Geometry check sheet. Reference: the model listing, model coordinates, mm. Face numbers are marked on the shaded views. Coordinates: 2 decimals unless noted, no trailing zeros. Write each loop counter-clockwise with the first axis right and the second up, starting at its lowest first coordinate (ties: lowest second). Pieces come first, ordered by that corner, then holes. Notation, with made-up numbers: (-18, 55) -> (3, 55) arc R23 cw to (3, 79) -> close; hole circle Ø8 at (21, 69.5). An arc over 180 degrees is marked (long way). Answer in a Markdown table with one row per item. Add a question column.
Q1. Section check A-A, the plane z = 5.25. Record the boundary of the cut face in (x, y), and give its area (3 significant figures).
Q2. Section check C-C, the plane x = 0.25. Record the boundary of the cut face in (y, z), and give its area (3 significant figures).
Q3. Gauge pin test, flat ends, axial feed: P1, Ø5, axis at x = 0, y = 0, coming from the -Z side; P2, Ø5, axis at x = 3, z = 6, coming from the -Y side; P3, Ø1.5, axis at x = 3, z = 3.5, coming from the -Y side. Record the tip position at first contact, or that the pin passes through.
Q4. Release check for a two-part mould opening along Y. For the marked faces 1, 2, 3 and 4 record: pulls with the +Y half, pulls with the -Y half, needs draft (parallel to the pull), parting line crosses it, or undercut.
Q5. Section check D-D, the plane x = -2.25. Record the boundary of the cut face in (y, z), and give its area (3 significant figures).
Q6. Thickness scan on line 1 (X direction, y = 0, z = 7.5); line 2 (X direction, y = 0, z = 3); line 3 (Z direction, x = 2.75, y = 2.25). Record the ranges inside material, lowest first.
Q7. Section check B-B, the plane y = 0. Record the boundary of the cut face in (x, z), and give its area (3 significant figures).
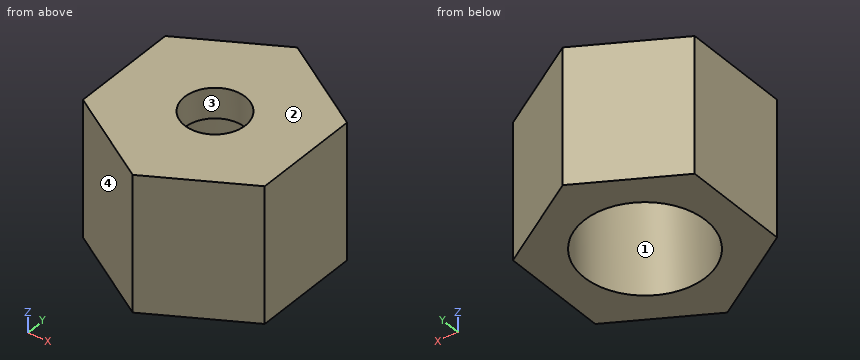
Autodesk Inventor part; units mm, degrees
ref_plane "YZ Plane" through (0, 0, 0) normal (1, 0, 0) x (0, 1, 0)
ref_plane "XZ Plane" through (0, 0, 0) normal (0, 1, 0) x (-1, 0, 0)
ref_plane "XY Plane" through (0, 0, 0) normal (0, 0, 1) x (1, 0, 0)
sketch "Sketch1" plane through (0, 0, 0) normal (0, 0, 1) x (1, 0, 0)
  line L0 (0, -6.9282) -> (-6, -3.4641)
  line L1 (-6, -3.4641) -> (-6, 3.4641)
  line L2 (-6, 3.4641) -> (0, 6.9282)
  line L3 (0, 6.9282) -> (6, 3.4641)
  line L4 (6, 3.4641) -> (6, -3.4641)
  line L5 (6, -3.4641) -> (0, -6.9282)
  line L6 (0, 0) -> (0, -16.3015)
  dimension "d0" = 12
extrude "Extrusion1" add sketch "Sketch1" along normal blind 9
hole "Hole1" at (0, 0, 0) direction (0, 0, 1) diameter 4 end through all counterbore diameter 8 counterbore depth 7
thread "Thread1"
properties part number "HUDSON-1-85"
Calculated:
| question | item | result |
|---|---|---|
| 1 | outline | (-6, -3.46) -> (0, -6.93) -> (6, -3.46) -> (6, 3.46) -> (0, 6.93) -> (-6, 3.46) -> close; hole circle Ø8 at (0, 0) |
| 1 | area | 74.4 mm² |
| 2 | outline | (-6.78, 0) -> (-3.99, 0) -> (-3.99, 7) -> (-1.98, 7) -> (-1.98, 9) -> (-6.78, 9) -> close; (1.98, 7) -> (3.99, 7) -> (3.99, 0) -> (6.78, 0) -> (6.78, 9) -> (1.98, 9) -> close |
| 2 | area | 58.3 mm² |
| 3 | P1 | stops at z = 7 |
| 3 | P2 | stops at y = -6.64 |
| 3 | P3 | stops at y = -5.63 |
| 4 | face 1 | undercut |
| 4 | face 2 | needs draft |
| 4 | face 3 | undercut |
| 4 | face 4 | pulls with the -Y half |
| 5 | outline | (-5.63, 0) -> (-3.31, 0) -> (-3.31, 7) -> (3.31, 7) -> (3.31, 0) -> (5.63, 0) -> (5.63, 9) -> (-5.63, 9) -> close |
| 5 | area | 55.0 mm² |
| 6 | line 1 | x = -6 to -2, 2 to 6 |
| 6 | line 2 | x = -6 to -4, 4 to 6 |
| 6 | line 3 | z = 7 to 9 |
| 7 | outline | (-6, 0) -> (-4, 0) -> (-4, 7) -> (-2, 7) -> (-2, 9) -> (-6, 9) -> close; (2, 7) -> (4, 7) -> (4, 0) -> (6, 0) -> (6, 9) -> (2, 9) -> close |
| 7 | area | 44.0 mm² |
